Geometry: final body of the model. Coordinates: model frame, mm. Face numbers are marked on the shaded views. A direction names the side the tool comes from. Round coordinates to 2 decimals unless told otherwise and drop trailing zeros. Write each loop counter-clockwise with the first axis right and the second up, starting at its lowest first coordinate (ties: lowest second). Pieces come first, ordered by that corner, then holes. Notation, with made-up numbers: (-27, -30) -> (-8, -30) arc R28 cw to (-8, -4) -> close; hole circle Ø11 at (21, 45.25). An arc over 180 degrees is marked (long way). One line per item, written item: value. Start each with the question number.
from build123d import *

# Parameters (mm, degrees)
SKETCH1_R           = 2.8
BOSS_EXTRUDE1_DEPTH = 4.5
SKETCH1_3_W         = 16.636354437
SKETCH1_3_H         = 16
BOSS_EXTRUDE2_DEPTH = 17.5
SKETCH2_W           = 9.45
SKETCH2_H           = 3.3
CUT_EXTRUDE1_DEPTH  = 17.636354437
CUT_EXTRUDE2_DEPTH  = 3.18
CUT_EXTRUDE3_REACH  = 19.5
SKETCH5_3_R         = 2.38125


with BuildPart() as part:
    # Sketch1 → Boss-Extrude1 (new body)
    with BuildSketch(Plane(origin=(0, 0, 0), x_dir=(1, 0, 0), z_dir=(0, 1, 0))):
        Polygon((30, 10), (-10, 10), (-10, -10), (6.636354437, -10), (20, -10), (30, -10), align=None)
        Circle(SKETCH1_R, mode=Mode.SUBTRACT)
        with Locations((20, 0)):
            Circle(SKETCH1_R, mode=Mode.SUBTRACT)
        Polygon((20, -10), (6.636354437, -10), (6.636354437, -26), align=None)
    extrude(amount=BOSS_EXTRUDE1_DEPTH)

    # Sketch1_3 → Boss-Extrude2 (add)
    with BuildSketch(Plane(origin=(0, 0, 0), x_dir=(1, 0, 0), z_dir=(0, 1, 0))):
        with Locations((-1.681822781, -18)):
            Rectangle(SKETCH1_3_W, SKETCH1_3_H)
    extrude(amount=BOSS_EXTRUDE2_DEPTH)

    # Sketch2 → Cut-Extrude1 (cut, through all)
    with BuildSketch(Plane(origin=(6.636354437, 0, 0), x_dir=(0, 0, -1), z_dir=(1, 0, 0))):
        with Locations((-18, 10)):
            Rectangle(SKETCH2_W, SKETCH2_H)
    extrude(amount=-CUT_EXTRUDE1_DEPTH, mode=Mode.SUBTRACT)

    # Sketch5 → Cut-Extrude2 (cut)
    with BuildSketch(Plane(origin=(0, 17.5, 0), x_dir=(1, 0, 0), z_dir=(0, 1, 0))):
        Polygon((0.701190454, -13.8725), (-4.064836018, -13.8725), (-6.447849254, -18), (-4.064836018, -22.1275), (0.701190454, -22.1275), (3.08420369, -18), align=None)
    extrude(amount=-CUT_EXTRUDE2_DEPTH, mode=Mode.SUBTRACT)

    # Sketch5_3 → Cut-Extrude3 (cut, up to next)
    with BuildSketch(Plane(origin=(0, 17.5, 0), x_dir=(1, 0, 0), z_dir=(0, 1, 0)), mode=Mode.PRIVATE) as cut_extrude3_sk1:
        with Locations((-1.681822782, -18)):
            Circle(SKETCH5_3_R)
    cut_extrude3_tool1 = extrude(cut_extrude3_sk1.sketch, amount=-CUT_EXTRUDE3_REACH, mode=Mode.PRIVATE) & part.part
    add(cut_extrude3_tool1.solids().sort_by_distance((-1.681823, 17.5, 18))[0], mode=Mode.SUBTRACT)


solid = part.part
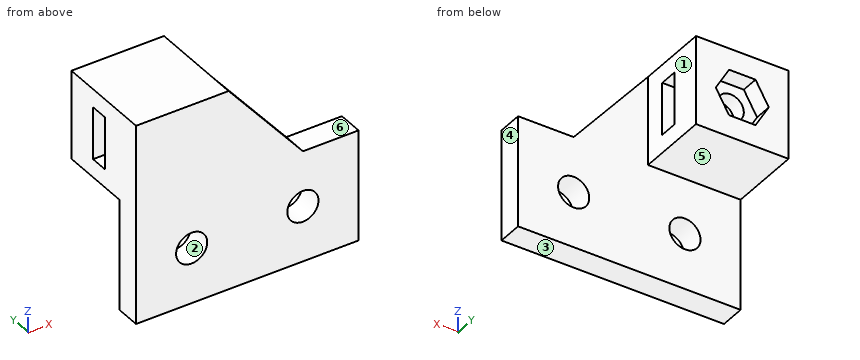
(1) Section query B-B (y = 3.25). Output: boundary loops of the cut face in (x, z), and give its area (3 significant figures).
(2) Set-up query: the marked faces 4, 5 and 6. Return all of +Z, -Z, +X, -X, +Y, -Y with unobstructed straight access to the full face (end or side cutting, diameter ignored); none if empty.
(3) Line query: probe 1 along X at (y, z) = (2.15, 0); probe 2 along Z at (x, y) = (0, 2.5); probe 3 along X at (y, z) = (13.4, 18). Output: solid intervals per line, ascending.
(4) Pull-direction query (Z, two-part tool) for the marked faces 1, 2 and 3; classes: pulls with the +Z half, pulls with the -Z half, needs draft (parallel to the pull), parting line crosses it, or undercut.
(5) Section query A-A (z = 0). Output: boundary loops of the cut face in (x, y), and give its area (3 significant figures).
(6) Section query D-D (x = 4). Output: boundary loops of the cut face in (y, z) (3 decimals), and give its area (3 significant figures).
(7) Pin query (flat end, axial travel): pin 1 (3.5 mm diameter, centred on x = -1.5, y = 9.5, fed in from -Z); pin 2 (5 mm diameter, centred on x = 25.5, y = 2.5, fed in from +Z); pin 3 (6 mm diameter, centred on y = 15, z = 20, fed in from +X). Return the tip coordinate at first contact, or that it passes through.
Results list:
1. outline: (-10, -10) -> (30, -10) -> (30, 10) -> (20, 10) -> (6.64, 26) -> (-10, 26) -> close; hole circle Ø5.6 at (0, 0); hole circle Ø5.6 at (20, 0)
1. area: 1,120 mm^2
2. face 4: +Z, -Z, +X, +Y, -Y
2. face 5: -Z, +X, -X, +Y
2. face 6: +Z, +X, +Y, -Y
3. probe 1: x = -10 to -2.8, 2.8 to 17.2, 22.8 to 30
3. probe 2: z = -10 to -2.8, 2.8 to 26
3. probe 3: x = -10 to -4.06, 0.7 to 6.64
4. face 1: needs draft
4. face 2: undercut
4. face 3: pulls with the -Z half
5. outline: (-10, 0) -> (-2.8, 0) -> (-2.8, 4.5) -> (-10, 4.5) -> close; (2.8, 0) -> (17.2, 0) -> (17.2, 4.5) -> (2.8, 4.5) -> close; (22.8, 0) -> (30, 0) -> (30, 4.5) -> (22.8, 4.5) -> close
5. area: 130 mm^2
6. outline: (0, -10) -> (4.5, -10) -> (4.5, 10) -> (17.5, 10) -> (17.5, 26) -> (0, 26) -> close; hole (8.35, 13.275) -> (11.65, 13.275) -> (11.65, 22.725) -> (8.35, 22.725) -> close
6. area: 339 mm^2
7. pin 1: stops at z = 10
7. pin 2: stops at z = 10
7. pin 3: stops at x = 6.64
